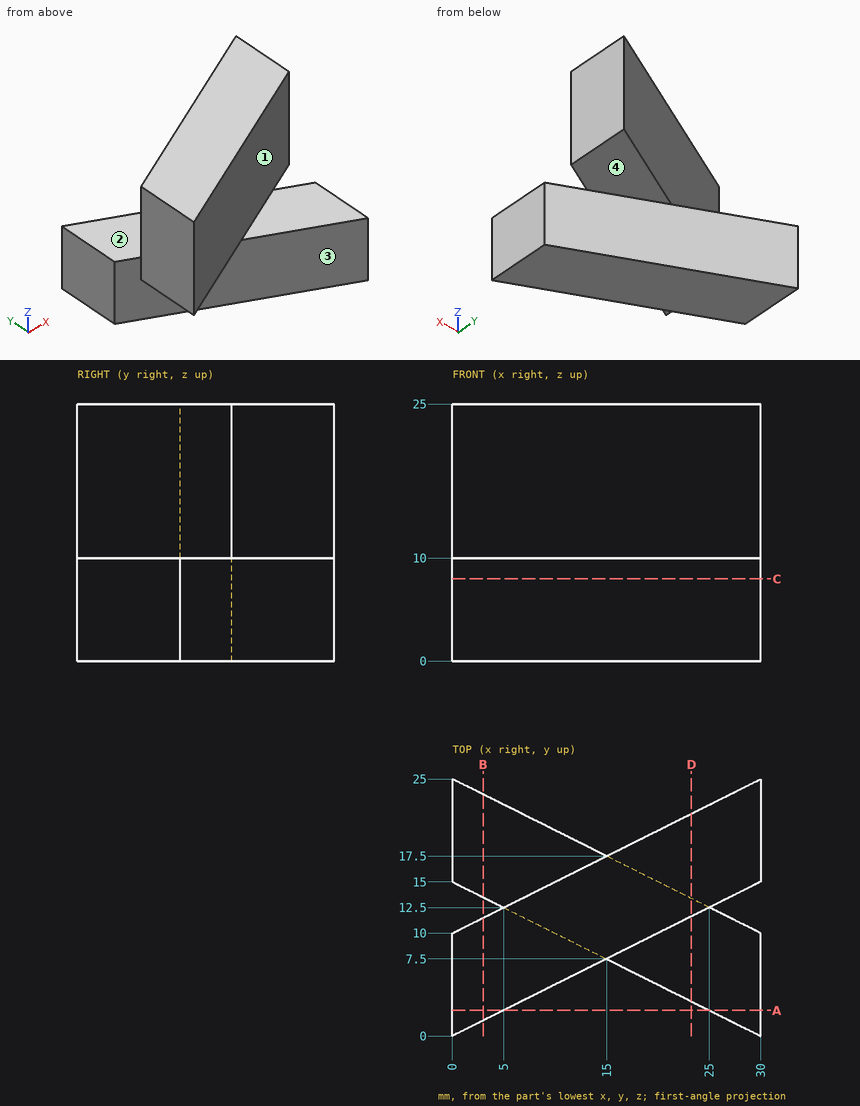
Source: three-view drawing plus pictorial views. Frame: mm from the lowest corner of the part. A direction names the side the tool comes from. Round coordinates to 2 decimals unless told otherwise and drop trailing zeros. Order: outer loops, then holes, each group sorted by start corner. A loop starts at its lowest first (then second) coordinate and runs counter-clockwise, first axis right, second up. Notation, with made-up numbers: (18.5, 5.5) -> (50.5, 5.5) arc R32 ccw to (50.5, 34.5) -> close; hole circle Ø1 at (-23.5, 16.5). An arc over 180 degrees is marked (long way). Use one line per item in the form item = value. Start each with the question number.
1. Cut plane D-D (x = 23.25). Return the cut outline in (y, z) (3 decimals).
2. Cut plane B-B (x = 3). Return the cut outline in (y, z).
3. Cut plane A-A (y = 2.5). Return the cut outline in (x, z).
4. Pin query (flat end, axial travel): pin 1 Ø10 at (x, y) = (23, 22) entering from -Z; pin 2 Ø6 at (x, y) = (11, 19) entering from +Z; pin 3 Ø2 at (y, z) = (3.5, 4) entering from -X. Return the tip coordinate at first contact, or that it passes through.
5. Cut plane C-C (z = 8). Return the cut outline in (x, y), then the cut area to 3 significant figures.
6. Line query: probe 1 along Z at (x, y) = (6.5, 20.5); probe 2 along Z at (x, y) = (4, 5.5); probe 3 along X at (y, z) = (6.25, 20.5). Output: solid intervals per line, ascending.
7. Reachability of the marked faces 1, 2, 3 and 4 from +Z, -Z, +X, -X, +Y, -Y: full face, straight path, thin tool, end or side. Return the list, or none.
Solution:
q1.outline = (3.375, 0) -> (13.375, 0) -> (13.375, 10) -> (21.625, 10) -> (21.625, 25) -> (11.625, 25) -> (11.625, 10) -> (3.375, 10) -> close
q2.outline = (1.5, 10) -> (11.5, 10) -> (11.5, 25) -> (1.5, 25) -> close; (13.5, 0) -> (23.5, 0) -> (23.5, 10) -> (13.5, 10) -> close
q3.outline = (0, 10) -> (5, 10) -> (5, 25) -> (0, 25) -> close; (25, 0) -> (30, 0) -> (30, 10) -> (25, 10) -> close
q4.pin_1 = 10
q4.pin_2 = 10
q4.pin_3 = 21
q5.outline = (0, 15) -> (30, 0) -> (30, 10) -> (0, 25) -> close
q5.area = 300 mm^2
q6.probe_1 = 0 to 10
q6.probe_2 = 10 to 25
q6.probe_3 = 0 to 12.5
q7.face_1 = +Z, +X, -Y
q7.face_2 = +Z, -X, +Y
q7.face_3 = -Z, -X, -Y
q7.face_4 = -Z, +X, +Y
